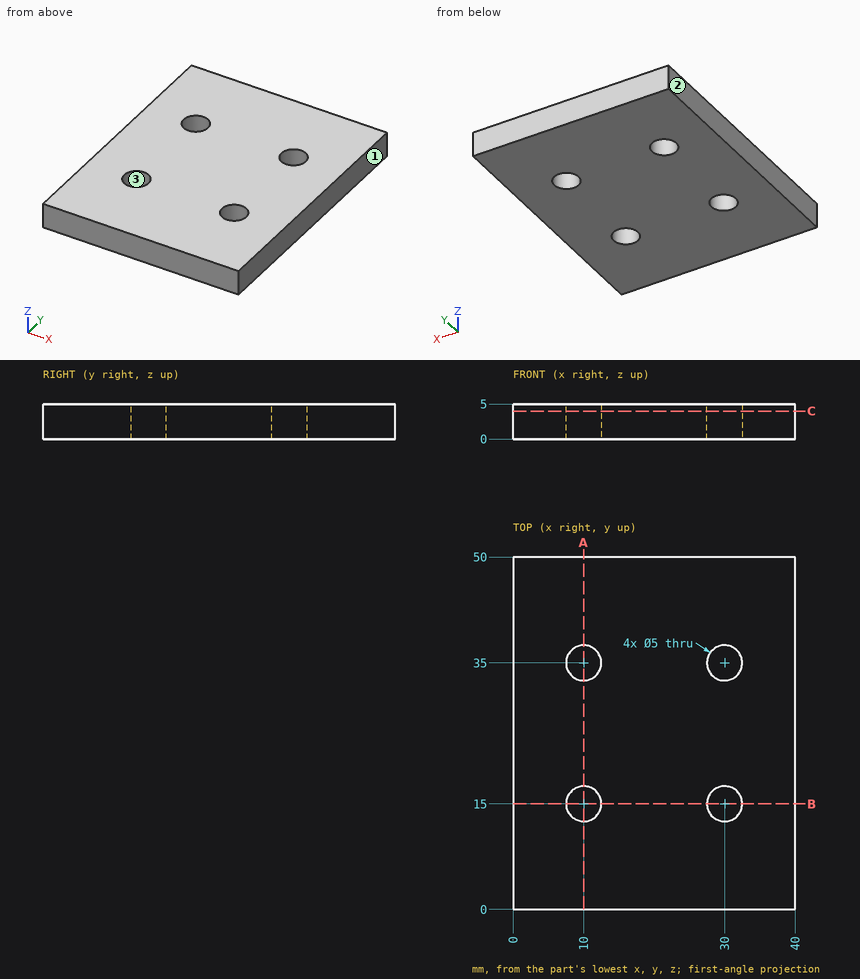
Print and shaded views of the part. All mm, measured from the part's lowest x, y and z. Give positions to 0.01 mm unless a question says otherwise; leave off trailing zeros. Order: outer loops, then holes, each group sorted by start corner. A loop starts at its lowest first (then second) coordinate and runs counter-clockwise, first axis right, second up. Notation, with made-up numbers: M 86,33 L 90,33 A20 ccw 90,56 Z; hole C 5,22.25 d5. An arc over 180 degrees is marked long. Use one line per item in the form item = value.
Q1. Pull direction X, two halves, no side cores. Call the marked faces 1, 2 and 3: released by +X, released by -X, zero draft, split by the parting line, or undercut.
Conclusion:
face_1 = released by +X
face_2 = released by -X
face_3 = undercut
Q2. Slice it at B-B, the plane y = 15. Write the cut outline in (x, z).
Conclusion:
outline = M 0,0 L 7.5,0 L 7.5,5 L 0,5 Z; M 12.5,0 L 27.5,0 L 27.5,5 L 12.5,5 Z; M 32.5,0 L 40,0 L 40,5 L 32.5,5 Z
Q3. Wall check: probe 1 along Y at (x, z) = (30, 2.65); probe 2 along Y at (x, z) = (9, 2.05); probe 3 along X at (y, z) = (36, 1.6). Give the ranges that are in metal, low to high.
Conclusion:
probe_1 = 0 to 12.5, 17.5 to 32.5, 37.5 to 50
probe_2 = 0 to 12.71, 17.29 to 32.71, 37.29 to 50
probe_3 = 0 to 7.71, 12.29 to 27.71, 32.29 to 40
Q4. Slice it at A-A, the plane x = 10. Write the cut outline in (y, z).
Conclusion:
outline = M 0,0 L 12.5,0 L 12.5,5 L 0,5 Z; M 17.5,0 L 32.5,0 L 32.5,5 L 17.5,5 Z; M 37.5,0 L 50,0 L 50,5 L 37.5,5 Z
Q5. Slice it at C-C, the plane z = 4. Write the cut outline in (x, y), and give its area (3 significant figures).
Conclusion:
outline = M 0,0 L 40,0 L 40,50 L 0,50 Z; hole C 10,15 d5; hole C 10,35 d5; hole C 30,15 d5; hole C 30,35 d5
area = 1,920 mm2
